Here's how the part is built. I have some questions about the finished solid (model axes, mm). Face numbers are marked on the shaded views. A direction names the side the tool comes from. Coordinates: 2 decimals unless noted, no trailing zeros. Write each loop counter-clockwise with the first axis right and the second up, starting at its lowest first coordinate (ties: lowest second). Pieces come first, ordered by that corner, then holes.
Item 1: For the marked faces 1 and 2, which set-ups out of +Z, -Z, +X, -X, +Y, -Y let a thin tool reach every point of the face, with its end or its side?
Item 2: If we section it at B-B (x = 0): Please give me the cut outline in (y, z).
Item 3: If we section it at C-C (z = 10.5): Please give me the cut outline in (x, y), then the cut area to 3 significant figures.
Item 4: If I drill on line 1 (Z direction, x = 1, y = 53.5); line 2 (Y direction, x = 16, z = 29.5); line 3 (Y direction, x = 35.5, z = 32.5), over which ranges is the centre line in solid material (lowest first)?
Item 5: If we section it at D-D (y = 38): Please give me the cut outline in (x, z).
Item 6: We'd pull the mould along Y, two halves only. Please class the marked faces 3, 4 and 5: +Y half, -Y half, draft (parallel to the pull), parting line (faces both ways), or undercut.
Item 7: I'm going to push flat-ended pins straight in: pin 1 Ø2.5 at (x, z) = (14.88, 7) entering from +Y; pin 2 Ø2.5 at (x, y) = (7.5, 105.51) entering from -Z; pin 3 Ø4.5 at (x, y) = (-17.51, 57.99) entering from +Z; pin 4 Ø18.5 at (x, z) = (43.5, 23) entering from +Y. Where does each tip first touch, or does it pass through?
Item 8: If we section it at A-A (z = 23): Count the separate pieces of the cut face and the enclosed holes in it, then the cut area to 3 significant figures.
from build123d import *

# Parameters (mm, degrees)
SKETCH023_R     = 1.7
PAD004_DEPTH    = 4
PAD005_DEPTH    = 2
SKETCH025_W     = 40
SKETCH025_H     = 3
PAD006_DEPTH    = 25
PAD007_DEPTH    = 5
SKETCH027_R     = 1.7
POCKET018_DEPTH = 10
SKETCH033_W     = 8.5
SKETCH033_H     = 16.5
POCKET021_DEPTH = 5


with BuildPart() as part:
    # Sketch023 → Pad004 (new body)
    with BuildSketch(Plane.XY):
        with BuildLine():
            Line((-52.5, 0), (-30.5, 0))
            Line((-30.5, 0), (30.5, 0))
            Line((30.5, 0), (52.5, 0))
            Line((52.5, 0), (52.5, 76.5))
            ThreePointArc((52.5, 76.5), (49.886128, 88.747449), (42.5, 98.86068))
            Line((42.5, 98.86068), (30, 110.04102))
            ThreePointArc((30, 110.04102), (0, 121.5), (-30, 110.04102))
            Line((-30, 110.04102), (-42.5, 98.86068))
            ThreePointArc((-42.5, 98.86068), (-49.886128, 88.747449), (-52.5, 76.5))
            Line((-52.5, 76.5), (-52.5, 0))
        make_face()
        with Locations((17.511522, 32.982072)):
            Circle(SKETCH023_R, mode=Mode.SUBTRACT)
        with Locations((17.511522, 47.982072)):
            Circle(SKETCH023_R, mode=Mode.SUBTRACT)
        with Locations((32.511522, 47.982072)):
            Circle(SKETCH023_R, mode=Mode.SUBTRACT)
        with Locations((32.511522, 32.982072)):
            Circle(SKETCH023_R, mode=Mode.SUBTRACT)
        with Locations((-7.5, 32.982072)):
            Circle(SKETCH023_R, mode=Mode.SUBTRACT)
        with Locations((-7.5, 47.982072)):
            Circle(SKETCH023_R, mode=Mode.SUBTRACT)
        with Locations((7.5, 47.982072)):
            Circle(SKETCH023_R, mode=Mode.SUBTRACT)
        with Locations((7.5, 32.982072)):
            Circle(SKETCH023_R, mode=Mode.SUBTRACT)
        with Locations((-32.511522, 32.982072)):
            Circle(SKETCH023_R, mode=Mode.SUBTRACT)
        with Locations((-32.511522, 47.982072)):
            Circle(SKETCH023_R, mode=Mode.SUBTRACT)
        with Locations((-17.511522, 47.982072)):
            Circle(SKETCH023_R, mode=Mode.SUBTRACT)
        with Locations((-17.511522, 32.982072)):
            Circle(SKETCH023_R, mode=Mode.SUBTRACT)
        with Locations((17.511522, 57.993594)):
            Circle(SKETCH023_R, mode=Mode.SUBTRACT)
        with Locations((17.511522, 72.993594)):
            Circle(SKETCH023_R, mode=Mode.SUBTRACT)
        with Locations((32.511522, 72.993594)):
            Circle(SKETCH023_R, mode=Mode.SUBTRACT)
        with Locations((32.511522, 57.993594)):
            Circle(SKETCH023_R, mode=Mode.SUBTRACT)
        with Locations((-7.5, 57.993594)):
            Circle(SKETCH023_R, mode=Mode.SUBTRACT)
        with Locations((-7.5, 72.993594)):
            Circle(SKETCH023_R, mode=Mode.SUBTRACT)
        with Locations((7.5, 72.993594)):
            Circle(SKETCH023_R, mode=Mode.SUBTRACT)
        with Locations((7.5, 57.993594)):
            Circle(SKETCH023_R, mode=Mode.SUBTRACT)
        with Locations((-32.511522, 57.993594)):
            Circle(SKETCH023_R, mode=Mode.SUBTRACT)
        with Locations((-32.511522, 72.993594)):
            Circle(SKETCH023_R, mode=Mode.SUBTRACT)
        with Locations((-17.511522, 72.993594)):
            Circle(SKETCH023_R, mode=Mode.SUBTRACT)
        with Locations((-17.511522, 57.993594)):
            Circle(SKETCH023_R, mode=Mode.SUBTRACT)
        with Locations((17.511522, 83.005116)):
            Circle(SKETCH023_R, mode=Mode.SUBTRACT)
        with Locations((17.511522, 98.005116)):
            Circle(SKETCH023_R, mode=Mode.SUBTRACT)
        with Locations((32.511522, 98.005116)):
            Circle(SKETCH023_R, mode=Mode.SUBTRACT)
        with Locations((32.511522, 83.005116)):
            Circle(SKETCH023_R, mode=Mode.SUBTRACT)
        with Locations((-7.5, 83.005116)):
            Circle(SKETCH023_R, mode=Mode.SUBTRACT)
        with Locations((-7.5, 98.005116)):
            Circle(SKETCH023_R, mode=Mode.SUBTRACT)
        with Locations((7.5, 98.005116)):
            Circle(SKETCH023_R, mode=Mode.SUBTRACT)
        with Locations((7.5, 83.005116)):
            Circle(SKETCH023_R, mode=Mode.SUBTRACT)
        with Locations((-32.511522, 83.005116)):
            Circle(SKETCH023_R, mode=Mode.SUBTRACT)
        with Locations((-32.511522, 98.005116)):
            Circle(SKETCH023_R, mode=Mode.SUBTRACT)
        with Locations((-17.511522, 98.005116)):
            Circle(SKETCH023_R, mode=Mode.SUBTRACT)
        with Locations((-17.511522, 83.005116)):
            Circle(SKETCH023_R, mode=Mode.SUBTRACT)
        with Locations((-7.5, 90.505116)):
            Circle(SKETCH023_R, mode=Mode.SUBTRACT)
        with Locations((-7.5, 105.505116)):
            Circle(SKETCH023_R, mode=Mode.SUBTRACT)
        with Locations((7.5, 105.505116)):
            Circle(SKETCH023_R, mode=Mode.SUBTRACT)
        with Locations((7.5, 90.505116)):
            Circle(SKETCH023_R, mode=Mode.SUBTRACT)
        with Locations((-24.827374, 3)):
            Circle(SKETCH023_R, mode=Mode.SUBTRACT)
        with Locations((-7.5, 3)):
            Circle(SKETCH023_R, mode=Mode.SUBTRACT)
        with Locations((7.5, 3)):
            Circle(SKETCH023_R, mode=Mode.SUBTRACT)
        with Locations((25.172626, 3)):
            Circle(SKETCH023_R, mode=Mode.SUBTRACT)
    extrude(amount=PAD004_DEPTH)

    # Sketch024 (on Face56 of Pad004) → Pad005 (join)
    with BuildSketch(Plane.XY.offset(4)):
        with BuildLine():
            Line((-52.5, 0), (-30.5, 0))
            Line((-30.5, 0), (-30.5, 6.5))
            Line((-30.5, 6.5), (30.5, 6.5))
            Line((30.5, 6.5), (30.5, 0))
            Line((30.5, 0), (52.5, 0))
            Line((52.5, 0), (52.5, 76.5))
            ThreePointArc((52.5, 76.5), (49.886128, 88.747449), (42.5, 98.86068))
            Line((42.5, 98.86068), (30, 110.04102))
            ThreePointArc((30, 110.04102), (0, 121.5), (-30, 110.04102))
            Line((-30, 110.04102), (-42.5, 98.86068))
            ThreePointArc((-42.5, 98.86068), (-49.886128, 88.747449), (-52.5, 76.5))
            Line((-52.5, 76.5), (-52.5, 0))
        make_face()
        with BuildLine():
            Line((-50.5, 2), (-50.5, 76.5))
            ThreePointArc((-40.126205, 98.86068), (-47.780263, 88.82493), (-50.5, 76.5))
            Line((-40.126205, 98.86068), (-26.907285, 110.04102))
            ThreePointArc((26.907285, 110.04102), (0, 119.500023), (-26.907285, 110.04102))
            Line((26.907285, 110.04102), (40.126205, 98.86068))
            ThreePointArc((50.5, 76.5), (47.780263, 88.82493), (40.126205, 98.86068))
            Line((50.5, 76.5), (50.5, 2.779082))
            Line((50.5, 2.779082), (35.5, 2.779082))
            ThreePointArc((32.5, 5.779082), (33.37868, 3.657761), (35.5, 2.779082))
            Line((32.5, 5.779082), (32.5, 9.5))
            Line((32.5, 9.5), (-32.5, 9.5))
            Line((-32.5, 9.5), (-32.5, 5))
            ThreePointArc((-35.5, 2), (-33.37868, 2.87868), (-32.5, 5))
            Line((-35.5, 2), (-50.5, 2))
        make_face(mode=Mode.SUBTRACT)
    extrude(amount=PAD005_DEPTH)

    # Sketch025 (on Face60 of Pad005) → Pad006 (join)
    with BuildSketch(Plane.XY.offset(6)):
        with BuildLine():
            Line((-52.5, 0), (-30.5, 0))
            Line((-30.5, 0), (-30.5, 6.5))
            Line((-32.5, 9.5), (-30.5, 6.5))
            Line((-32.5, 9.5), (-32.5, 5))
            ThreePointArc((-35.5, 2), (-33.37868, 2.87868), (-32.5, 5))
            Line((-35.5, 2), (-50.5, 2))
            Line((-50.5, 2), (-52.5, 2))
            Line((-52.5, 2), (-52.5, 0))
        make_face()
        with Locations((0, 8)):
            Rectangle(SKETCH025_W, SKETCH025_H)
        with BuildLine():
            Line((30.5, 6.5), (30.5, 0))
            Line((30.5, 0), (52.5, 0))
            Line((52.5, 2.779082), (52.5, 0))
            Line((50.5, 2.779082), (52.5, 2.779082))
            Line((50.5, 2.779082), (35.5, 2.779082))
            ThreePointArc((32.5, 5.779082), (33.37868, 3.657761), (35.5, 2.779082))
            Line((32.5, 5.779082), (32.5, 9.5))
            Line((30.5, 6.5), (32.5, 9.5))
        make_face()
    extrude(amount=PAD006_DEPTH)

    # Sketch026 (on Face102 of Pad006) → Pad007 (join)
    with BuildSketch(Plane.XY.offset(31)):
        with BuildLine():
            Line((-52.5, 0), (-30.5, 0))
            Line((-30.5, 0), (-30.5, 6.5))
            Line((-30.5, 6.5), (30.5, 6.5))
            Line((30.5, 6.5), (30.5, 0))
            Line((30.5, 0), (52.5, 0))
            Line((52.5, 2.779082), (52.5, 0))
            Line((50.5, 2.779082), (52.5, 2.779082))
            Line((50.5, 2.779082), (35.5, 2.779082))
            ThreePointArc((32.5, 5.779082), (33.37868, 3.657761), (35.5, 2.779082))
            Line((32.5, 5.779082), (32.5, 9.5))
            Line((32.5, 9.5), (-32.5, 9.5))
            Line((-32.5, 9.5), (-32.5, 5))
            ThreePointArc((-35.5, 2), (-33.37868, 2.87868), (-32.5, 5))
            Line((-35.5, 2), (-50.5, 2))
            Line((-52.5, 2), (-50.5, 2))
            Line((-52.5, 0), (-52.5, 2))
        make_face()
    extrude(amount=PAD007_DEPTH)

    # Sketch027 (on Face114 of Pad007) → Pocket018 (cut)
    with BuildSketch(Plane(origin=(0, 9.5, 0), x_dir=(-1, 0, 0), z_dir=(0, 1, 0))):
        with Locations((-14.881968, 23)):
            Circle(SKETCH027_R)
        with Locations((0, 23)):
            Circle(SKETCH027_R)
        with Locations((15.118032, 23)):
            Circle(SKETCH027_R)
        with Locations((15.118032, 7)):
            Circle(SKETCH027_R)
        with Locations((0, 7)):
            Circle(SKETCH027_R)
        with Locations((-14.881968, 7)):
            Circle(SKETCH027_R)
    extrude(amount=-POCKET018_DEPTH, mode=Mode.SUBTRACT)

    # Sketch033 (on Face72 of Pocket018) → Pocket021 (cut)
    with BuildSketch(Plane.XY.offset(4)):
        with Locations((-44.25, 53.25)):
            Rectangle(SKETCH033_W, SKETCH033_H)
    extrude(amount=-POCKET021_DEPTH, mode=Mode.SUBTRACT)


solid = part.part
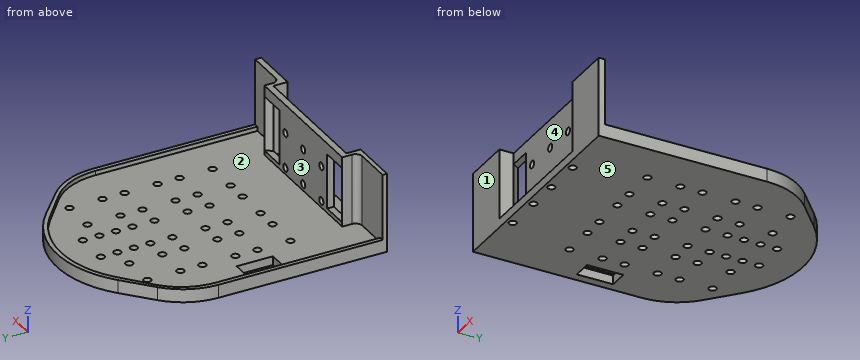
Answer list:
1. face 1: +Z, -Z, +X, -X, -Y
1. face 2: +Z
2. outline: (0, 0) - (121.5, 0) - (121.5, 6) - (119.5, 6) - (119.5, 4) - (9.5, 4) - (9.5, 5.3) - (6.5, 5.3) - (6.5, 4) - (0, 4) - close; (6.5, 8.7) - (9.5, 8.7) - (9.5, 21.3) - (6.5, 21.3) - close; (6.5, 24.7) - (9.5, 24.7) - (9.5, 36) - (6.5, 36) - close
3. outline: (-52.5, 0) - (-30.5, 0) - (-30.5, 6.5) - (-32.5, 9.5) - (-32.5, 5) arc R3 cw to (-35.5, 2) - (-52.5, 2) - close; (-20, 6.5) - (20, 6.5) - (20, 9.5) - (-20, 9.5) - close; (30.5, 0) - (52.5, 0) - (52.5, 2.78) - (35.5, 2.78) arc R3 cw to (32.5, 5.78) - (32.5, 9.5) - (30.5, 6.5) - close
3. area: 251 mm2
4. line 1: z = 0 to 4
4. line 2: y = 6.5 to 9.5
4. line 3: y = 0 to 2.78
5. outline: (-52.5, 0) - (52.5, 0) - (52.5, 6) - (50.5, 6) - (50.5, 4) - (-50.5, 4) - (-50.5, 6) - (-52.5, 6) - close
6. face 3: undercut
6. face 4: -Y half
6. face 5: draft
7. pin 1: stops at y = 119.22
7. pin 2: passes through
7. pin 3: stops at z = 4
7. pin 4: stops at y = 3.05
8. separate pieces: 6
8. enclosed holes: 0
8. area: 221 mm2
